Geometry check sheet. Reference: drawing and pictorial views, mm from the part's lowest x, y, z. A direction names the side the tool comes from. Round coordinates to 2 decimals unless told otherwise and drop trailing zeros. Write each loop counter-clockwise with the first axis right and the second up, starting at its lowest first coordinate (ties: lowest second). Pieces come first, ordered by that corner, then holes. Notation, with made-up numbers: M -5,15 L 47,15 A15 cw 47,25 Z; hole C 39,37.5 d8. An arc over 180 degrees is marked long. One line per item, written item: value. Start each with the question number.
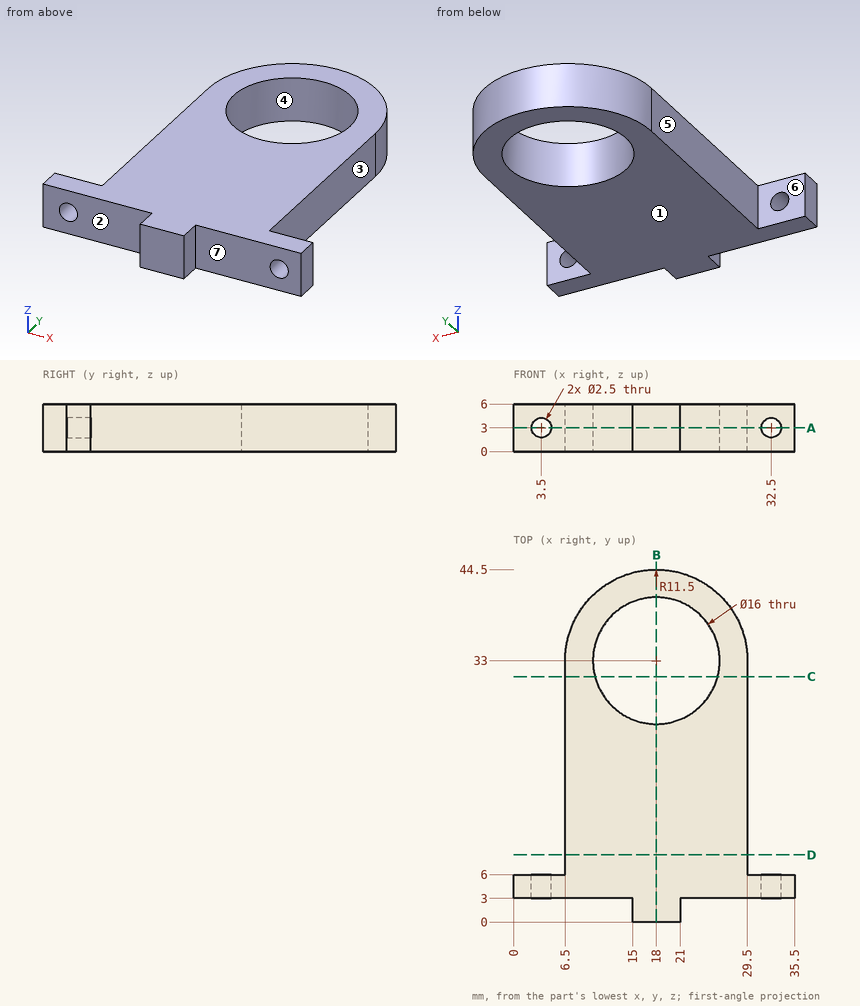
1) Cross-section at C-C (y = 31). Record the boundary of the cut face in (x, z), then the cut area to 3 significant figures.
2) Cross-section at B-B (x = 18). Record the boundary of the cut face in (y, z).
3) Access from +Z, -Z, +X, -X, +Y, -Y to the whole of each face (thin tool, end or side, straight path). Record for the marked faces 1, 2 and 3.
4) Gauge pin test, flat ends, axial feed: pin 1 Ø3 at (x, z) = (3.5, 3) entering from -Y; pin 2 Ø13 at (x, y) = (18, 33) entering from -Z; pin 3 Ø1.5 at (y, z) = (35, 1.5) entering from -X; pin 4 Ø3 at (y, z) = (19, 2) entering from -X. Record the tip position at first contact, or that the pin passes through.
5) Cross-section at D-D (y = 8.5). Record the boundary of the cut face in (x, z), then the cut area to 3 significant figures.
6) Cross-section at A-A (z = 3). Record the boundary of the cut face in (x, y).
7) Mould release check, pull along Y, two halves, no side actions. Record for the marked faces 4, 5, 6 and 7: pulls with the +Y half, pulls with the -Y half, needs draft (parallel to the pull), parting line crosses it, or undercut.
8) Thickness scan on line 1 (X direction, y = 5.1, z = 3); line 2 (Z direction, x = 32.5, y = 4.75); line 3 (Y direction, x = 18, z = 1.5). Record the ranges inside material, lowest first.
Results below:
1. outline: M 6.5,0 L 10.25,0 L 10.25,6 L 6.5,6 Z; M 25.75,0 L 29.5,0 L 29.5,6 L 25.75,6 Z
1. area: 45.0 mm²
2. outline: M 0,0 L 25,0 L 25,6 L 0,6 Z; M 41,0 L 44.5,0 L 44.5,6 L 41,6 Z
3. face 1: -Z, +X, -X, +Y, -Y
3. face 2: +Z, -Z, -X, -Y
3. face 3: +Z, -Z, +X, +Y
4. pin 1: stops at y = 3
4. pin 2: passes through
4. pin 3: stops at x = 6.57
4. pin 4: stops at x = 6.5
5. outline: M 6.5,0 L 29.5,0 L 29.5,6 L 6.5,6 Z
5. area: 138 mm²
6. outline: M 0,3 L 2.25,3 L 2.25,6 L 0,6 Z; M 4.75,3 L 15,3 L 15,0 L 21,0 L 21,3 L 31.25,3 L 31.25,6 L 29.5,6 L 29.5,33 A11.5 ccw 6.5,33 L 6.5,6 L 4.75,6 Z; M 33.75,3 L 35.5,3 L 35.5,6 L 33.75,6 Z; hole C 18,33 d16
7. face 4: undercut
7. face 5: needs draft
7. face 6: pulls with the +Y half
7. face 7: pulls with the -Y half
8. line 1: x = 0 to 2.25, 4.75 to 31.25, 33.75 to 35.5
8. line 2: z = 0 to 1.75, 4.25 to 6
8. line 3: y = 0 to 25, 41 to 44.5
